```python
from build123d import *

# Parameters (mm, degrees)
F0_W     = 66
F0_H     = 87
F1_DEPTH = 13.5
F3_DEPTH = 70
F4_DEPTH = 66


with BuildPart() as f1:
    # F0 (on Front) → F1 (new body, symmetric)
    with BuildSketch(Plane.XZ):
        Rectangle(F0_W, F0_H)
    extrude(amount=F1_DEPTH, both=True)

    # F2 (on face) → F3 (cut)
    with BuildSketch(Plane(origin=(-33, 0, 0), x_dir=(0, -1, 0), z_dir=(-1, 0, 0))):
        Polygon((13.5, 35.5), (13.5, 43.5), (-13.5, 43.5), (-13.5, 23.5), align=None)
    extrude(amount=-F3_DEPTH, mode=Mode.SUBTRACT)

    # F2 (on face) → F4 (join)
    with BuildSketch(Plane(origin=(-33, 0, 0), x_dir=(0, -1, 0), z_dir=(-1, 0, 0))):
        with BuildLine():
            ThreePointArc((16, 33), (14.232233047, 33.732233047), (13.5, 35.5))
            Line((13.5, 35.5), (13.5, 33))
            Line((13.5, 33), (16, 33))
        make_face()
        with BuildLine():
            ThreePointArc((18.0551601423, 36.9234875445), (15.2543125172, 37.8861999451), (13.5, 35.5))
            ThreePointArc((13.5, 35.5), (14.232233047, 33.732233047), (16, 33))
            ThreePointArc((16, 33), (17.767766953, 33.732233047), (18.5, 35.5))
            ThreePointArc((18.5, 35.5), (18.3861999451, 36.2456874828), (18.0551601423, 36.9234875445))
        make_face()
        with BuildLine():
            Line((18.0551601423, 36.9234875445), (13.5, 43.5))
            Line((13.5, 43.5), (13.5, 35.5))
            ThreePointArc((13.5, 35.5), (15.2543125172, 37.8861999451), (18.0551601423, 36.9234875445))
        make_face()
    extrude(amount=-F4_DEPTH)


solid = f1.part
```
Source: CAD feature listing. Evaluate the final solid. Frame: model axes, mm. A direction names the side the tool comes from. Coordinates: 2 decimals unless noted, no trailing zeros. Loops run counter-clockwise (first coordinate to the right, second up) from the corner with the lowest first, then second, coordinate; pieces in that order, holes last. Notation, with made-up numbers: M 21.25,7.25 L 48.25,7.25 A17 ccw 48.25,28.25 Z; hole C 25,65 d11. An arc over 180 degrees is marked long. Use CSV: the item, a comma, the result in double quotes.
(1) Cut plane A-A on x = 11. Return loops of the section in (y, z), and give its area (3 significant figures).
Answers follow:
outline,"M -18.06,36.92 A2.5 ccw -16,33 L -13.5,33 L -13.5,-43.5 L 13.5,-43.5 L 13.5,23.5 L -13.5,35.5 L -13.5,43.5 Z"
area,"2,000 mm²"
(2) Cut plane B-B on z = -26.5. Return loops of the section in (x, y), and give its area (3 significant figures).
Answers follow:
outline,"M -33,-13.5 L 33,-13.5 L 33,13.5 L -33,13.5 Z"
area,"1,780 mm²"
(3) Cut plane C-C on y = 11. Return loops of the section in (x, z).
Answers follow:
outline,"M -33,-43.5 L 33,-43.5 L 33,24.61 L -33,24.61 Z"
(4) Reachability of faces 1 (the face through (-0.462, -15.809, 40.166)), 2 (the face through (0, -13.5, -5)), 3 (the face through (0, -13.5, 40)) from +Z, -Z, +X, -X, +Y, -Y: full face, straight path, thin tool, end or side. Return the list, or none.
Answers follow:
face 1,"+Z, +X, -X, -Y"
face 2,"-Z, +X, -X, -Y"
face 3,"+Z, +X, -X, +Y"
(5) Contact query for flat-ended pins moving along their axis: pin 1 (4 mm diameter, centred on x = -15, z = 39.5, fed in from +Y); pin 2 (1 mm diameter, centred on x = 20, z = 26.5, fed in from -Y); pin 3 (1 mm diameter, centred on x = -16, y = -1, fed in from +Z). Output: stop coordinate, or through.
Answers follow:
pin 1,"y = -13.5"
pin 2,"y = -13.5"
pin 3,"z = 30.17"
(6) Line query: line 1 (Y direction, x = 11, z = 12); line 2 (Z direction, x = 5.5, y = -7); line 3 (Z direction, x = 3, y = -11). Output: solid intervals per line, ascending. Write a range as [from, to].
Answers follow:
line 1,"[-13.5, 13.5]"
line 2,"[-43.5, 32.61]"
line 3,"[-43.5, 34.39]"
